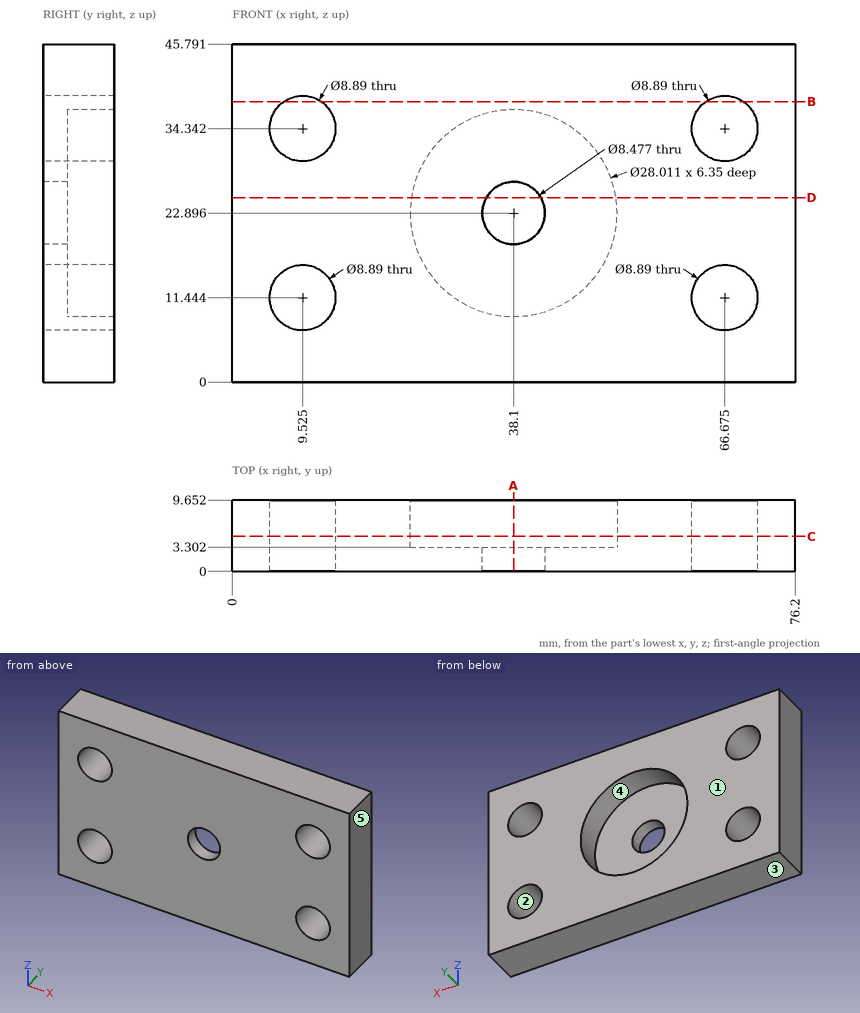
For this review, use the dimensioned drawing (mm, ordinates from the lowest corner) and the shaded views. A direction names the side the tool comes from. Round coordinates to 2 decimals unless told otherwise and drop trailing zeros. Order: outer loops, then holes, each group sorted by start corner. A loop starts at its lowest first (then second) coordinate and runs counter-clockwise, first axis right, second up. Notation, with made-up numbers: (29.5, 42) -> (41.5, 42) arc R16 ccw to (41.5, 60) -> close; hole circle Ø6 at (-11, 81). An arc over 180 degrees is marked (long way). Use CSV: the item, a comma, the result in double quotes. Start each with the question number.
(1) Consider section B-B on z = 38. Write out the cut boundary in (x, y), and give its area (3 significant figures).
(2) Consider section A-A on x = 38.1. Write out the cut boundary in (y, z) (1 decimal), and give its area (3 significant figures).
(3) Wall thickness on probe 1 along Z at (x, y) = (38.1, 8); probe 2 along X at (y, z) = (1.75, 9); probe 3 along X at (y, z) = (8.5, 7.5) (1 decimal): over which ranges is each line inside the solid? List them lowest first. Write a range as from..to.
(4) Consider section D-D on z = 25. Write out the cut boundary in (x, y).
(5) Mouldability with a two-part tool opening along Z and no side actions: class the marked faces 1, 2 and 3 as pulls with the +Z half, pulls with the -Z half, needs draft (parallel to the pull), parting line crosses it, or undercut.
(6) Insertion check: pin 1 (8.5 mm diameter, centred on x = 44, z = 20.5, fed in from +Y); pin 2 (7 mm diameter, centred on x = 38.1, z = 22.9, fed in from -Y). Each pin has a flat end and moves straight along its axis. Give the tip position at first contact, or say it passes through.
(7) Consider section C-C on y = 4.75. Write out the cut boundary in (x, z) (1 decimal).
(8) Tool access review of the marked faces 4 and 5: name each direction out of +Z, -Z, +X, -X, +Y, -Y from which nothing blocks a thin tool from reaching the whole face with its end or side.
Responses:
1,outline,"(0, 0) -> (7, 0) -> (7, 9.65) -> (0, 9.65) -> close; (12.05, 0) -> (64.15, 0) -> (64.15, 9.65) -> (12.05, 9.65) -> close; (69.2, 0) -> (76.2, 0) -> (76.2, 9.65) -> (69.2, 9.65) -> close"
1,area,"638 mm²"
2,outline,"(0, 0) -> (9.7, 0) -> (9.7, 8.9) -> (3.3, 8.9) -> (3.3, 18.7) -> (0, 18.7) -> close; (0, 27.1) -> (3.3, 27.1) -> (3.3, 36.9) -> (9.7, 36.9) -> (9.7, 45.8) -> (0, 45.8) -> close"
2,area,"236 mm²"
3,probe 1,"0..8.89, 36.9..45.79"
3,probe 2,"0..5.81, 13.24..62.96, 70.39..76.2"
3,probe 3,"0..7.5, 11.6..64.6, 68.7..76.2"
4,outline,"(0, 0) -> (34.42, 0) -> (34.42, 3.3) -> (24.25, 3.3) -> (24.25, 9.65) -> (0, 9.65) -> close; (41.78, 0) -> (76.2, 0) -> (76.2, 9.65) -> (51.95, 9.65) -> (51.95, 3.3) -> (41.78, 3.3) -> close"
5,face 1,"needs draft"
5,face 2,"undercut"
5,face 3,"pulls with the -Z half"
6,pin 1,"y = 3.3"
6,pin 2,"through"
7,outline,"(0, 0) -> (76.2, 0) -> (76.2, 45.8) -> (0, 45.8) -> close; hole circle Ø8.9 at (9.5, 11.4); hole circle Ø8.9 at (9.5, 34.3); hole circle Ø28 at (38.1, 22.9); hole circle Ø8.9 at (66.7, 11.4); hole circle Ø8.9 at (66.7, 34.3)"
8,face 4,"+Y"
8,face 5,"+Z, -Z, +X, +Y, -Y"
